Can you work these out from the model? Positions are in its coordinate system, mm. A direction names the side the tool comes from. Coordinates: 2 decimals unless noted, no trailing zeros. Order: outer loops, then holes, each group sorted by start corner. A loop starts at its lowest first (then second) coordinate and runs counter-clockwise, first axis right, second up. Notation, with made-up numbers: M 47,30.25 L 52,30.25 A3 cw 52,34.25 Z; hole C 43,59.5 d6. An arc over 180 degrees is marked long. Answer as CSV lines item,"result". Start each with the question number.
1. If we section it at A-A (x = 45.5): List the corners of the cut face in (y, z) for me.
2. If we mould it in two halves opening along Y, with no side actions, what happens to faces 3 (the face through (188, -36.112, 9)), 4 (the face through (331.238, 154, 10)), 5 (the face through (188, 192.488, 9)), 6 (the face through (188, 80, 0))? For each: released by +Y, released by -Y, zero draft, split by the parting line, or undercut.
3. I need wall thicknesses on line 1 along Y through (x, z) = (381, 10); line 2 along Y through (x, z) = (37.5, 13). Which ranges of each line are inside material? Lowest first, please. Write a range as from..to.
4. On a 3-axis mill with a long thin cutter (end or side, diameter ignored), from which of +Z, -Z, +X, -X, +Y, -Y can I reach the whole of each face in a straight line? I mean faces 1 (the face through (341, 160.688, 10)), 2 (the face through (-23.613, 77, 9)). Say none if no direction works.
```python
from build123d import *

# Parameters (mm, degrees)
SKETCH1_W           = 428.225
SKETCH1_H           = 228.6
SKETCH1_R           = 3.3655
SKETCH1_R_2         = 12.192
BOSS_EXTRUDE1_DEPTH = 19.05
SKETCH2_W           = 19.75
SKETCH2_H           = 12.6
CUT_EXTRUDE1_DEPTH  = 449.470305943


with BuildPart() as part:
    # Sketch1 → Boss-Extrude1 (new body)
    with BuildSketch(Plane.XY):
        with Locations((190.5, 78.1875)):
            Rectangle(SKETCH1_W, SKETCH1_H)
        with Locations(Location((0, -23.6125, 0), (0, 0, 180))):
            Circle(SKETCH1_R, mode=Mode.SUBTRACT)
        with Locations(Location((381, -23.6125, 0), (0, 0, 180))):
            Circle(SKETCH1_R, mode=Mode.SUBTRACT)
        with Locations(Location((381, 179.9875, 0), (0, 0, 180))):
            Circle(SKETCH1_R, mode=Mode.SUBTRACT)
        with Locations(Location((0, 179.9875, 0), (0, 0, 180))):
            Circle(SKETCH1_R, mode=Mode.SUBTRACT)
        with Locations(Location((39.8875, 154.3875, 0), (0, 0, 180))):
            Circle(SKETCH1_R_2, mode=Mode.SUBTRACT)
    extrude(amount=BOSS_EXTRUDE1_DEPTH)

    # Sketch2 → Cut-Extrude1 (cut, through all)
    with BuildSketch(Plane.XY.offset(19.05)):
        with Locations((341.1125, 154.3875)):
            Rectangle(SKETCH2_W, SKETCH2_H)
    extrude(amount=-CUT_EXTRUDE1_DEPTH, mode=Mode.SUBTRACT)


solid = part.part
```
Solved:
1,outline,"M -36.11,0 L 143.56,0 L 143.56,19.05 L -36.11,19.05 Z; M 165.21,0 L 192.49,0 L 192.49,19.05 L 165.21,19.05 Z"
2,face 3,"released by -Y"
2,face 4,"undercut"
2,face 5,"released by +Y"
2,face 6,"zero draft"
3,line 1,"-36.11..-26.98, -20.25..176.62, 183.35..192.49"
3,line 2,"-36.11..142.43, 166.34..192.49"
4,face 1,"+Z, -Z"
4,face 2,"+Z, -Z, -X, +Y, -Y"
